from build123d import *

# Parameters (mm, degrees)
SKETCH3_R                                           = 21
CUT_EXTRUDE1_DEPTH                                  = 12
FILLET1_R                                           = 1
FILLET2_R                                           = 2
CBORE_FOR_M6_HEX_SOCKET_HEAD_CAP_SCREW1_D           = 6.6
CBORE_FOR_M6_HEX_SOCKET_HEAD_CAP_SCREW1_CBORE_D     = 11
CBORE_FOR_M6_HEX_SOCKET_HEAD_CAP_SCREW1_CBORE_DEPTH = 6.4


with BuildPart() as part:
    # Sketch1 → Revolve1 (revolve)
    with BuildSketch(Plane.XY, mode=Mode.PRIVATE) as revolve1_sk:
        Polygon((0, 0), (0, 62), (5, 62), (5, 41), (16, 41), (16, 0), align=None)
    revolve(revolve1_sk.sketch.rotate(Axis((16, 0, 0), (-1, 0, 0)), 90), axis=Axis((16, 0, 0), (-1, 0, 0)))

    # Sketch3 → Cut-Extrude1 (cut)
    with BuildSketch(Plane.ZY):
        Circle(SKETCH3_R)
    extrude(amount=-CUT_EXTRUDE1_DEPTH, mode=Mode.SUBTRACT)

    # Fillet1
    fillet1_edges = [part.edges().sort_by_distance(p)[0] for p in [
        (12, 0, -21),
    ]]
    fillet(fillet1_edges, radius=FILLET1_R)

    # Fillet2
    fillet2_edges = [part.edges().sort_by_distance(p)[0] for p in [
        (16, 0, 41),
    ]]
    fillet(fillet2_edges, radius=FILLET2_R)

    # CBORE for M6 Hex Socket Head Cap Screw1 (through all)
    with Locations(Plane(origin=(16, 0, 0), x_dir=(0, 0, -1), z_dir=(1, 0, 0))):
        with Locations((0, -32), (32, 0), (0, 32), (-32, 0)):
            CounterBoreHole(CBORE_FOR_M6_HEX_SOCKET_HEAD_CAP_SCREW1_D / 2, CBORE_FOR_M6_HEX_SOCKET_HEAD_CAP_SCREW1_CBORE_D / 2, CBORE_FOR_M6_HEX_SOCKET_HEAD_CAP_SCREW1_CBORE_DEPTH)


solid = part.part
Input: part model. Units: mm. Frame: model coordinates. A direction names the side the tool comes from. Round coordinates to 2 decimals unless told otherwise and drop trailing zeros. Order: outer loops, then holes, each group sorted by start corner. A loop starts at its lowest first (then second) coordinate and runs counter-clockwise, first axis right, second up. Notation, with made-up numbers: (-30, 6) - (2, 6) arc R25 cw to (2, 18) - close; hole circle Ø11 at (51.25, -30). An arc over 180 degrees is marked (long way). Answer as a JSON object with one key per item and string values. Group by question number.
(1) Cut plane D-D (y = 48). Return loops of the section in (x, z), then the cut area to 3 significant figures.
(2) Draft query along Z for faces 1 (the face through (5, 40, -13)), 2 (the face through (4.73, 0.99, 35.15)), 3 (the face through (9.563, 15.703, -37.874)). Return one class per face: released by +Z, released by -Z, zero draft, split by the parting line, or undercut.
(3) Reachability of faces 4 (the face through (9.6, 0, -36)), 5 (the face through (16, -1, 1)), 6 (the face through (12, 0, 0)) from +Z, -Z, +X, -X, +Y, -Y: full face, straight path, thin tool, end or side. Return the list, or none.
(4) Pin query (flat end, axial travel): P1, Ø9, axis at y = -0.5, z = -32, coming from the +X side; P2, Ø5.5, axis at y = -32, z = 0, coming from the -X side; P3, Ø3, axis at x = 8, z = -4.5, coming from the -Y side; P4, Ø6, axis at x = 12.5, z = 2.5, coming from the +Y side. Return the tip coordinate at first contact, or that it passes through.
(5) Cut plane A-A (z = 0). Count the separate pieces of the cut face and the enclosed holes in it, then the cut area to 3 significant figures.
(6) Cut plane C-C (x = 6.5). Return loops of the section in (y, z).
(7) Material intervals for probe 1 along Y at (x, z) = (7.25, 0); probe 2 along Y at (x, z) = (11, 0); probe 3 along Z at (x, y) = (1, 46.5), sorted ascending. Write a range as from..to.
Here are the results:
{
 "1": {"outline": "(0, -39.24) - (5, -39.24) - (5, 39.24) - (0, 39.24) - close", "area": "392 mm^2"},
 "2": {"face 1": "zero draft", "face 2": "undercut", "face 3": "split by the parting line"},
 "3": {"face 4": "+X", "face 5": "+Z, -Z, +X, +Y, -Y", "face 6": "-X"},
 "4": {"P1": "stops at x = 9.6", "P2": "passes through", "P3": "stops at y = -40.89", "P4": "stops at y = 41"},
 "5": {"separate pieces": "3", "enclosed holes": "0", "area": "749 mm^2"},
 "6": {"outline": "circle Ø82 at (0, 0); hole circle Ø6.6 at (-32, 0); hole circle Ø42 at (0, 0); hole circle Ø6.6 at (0, -32); hole circle Ø6.6 at (0, 32); hole circle Ø6.6 at (32, 0)"},
 "7": {"probe 1": "y = -41..-35.3, -28.7..-21, 21..28.7, 35.3..41", "probe 2": "y = -41..-37.5, -26.5..-21, 21..26.5, 37.5..41", "probe 3": "z = -41.01..41.01"}
}
